```python
from build123d import *

# Parameters (mm, degrees)
SKETCH1_W           = 15
SKETCH1_H           = 4
BOSS_EXTRUDE1_DEPTH = 4.5
SKETCH2_W           = 6
SKETCH2_H           = 3
CUT_EXTRUDE1_DEPTH  = 4.5
SKETCH3_W           = 0.5
SKETCH3_H           = 4.5
CUT_EXTRUDE2_DEPTH  = 9.5
SKETCH4_W           = 0.5
SKETCH4_H           = 4.5
CUT_EXTRUDE3_DEPTH  = 9.5
SKETCH6_W           = 14
SKETCH6_H           = 0.5
CUT_EXTRUDE5_DEPTH  = 9.5


with BuildPart() as part:
    # Sketch1 → Boss-Extrude1 (new body)
    with BuildSketch(Plane(origin=(0, 0, 0), x_dir=(1, 0, 0), z_dir=(0, 1, 0))):
        with Locations((7.5, 2)):
            Rectangle(SKETCH1_W, SKETCH1_H)
    extrude(amount=BOSS_EXTRUDE1_DEPTH)

    # Sketch2 → Cut-Extrude1 (cut)
    with BuildSketch(Plane(origin=(0, 4.5, 0), x_dir=(1, 0, 0), z_dir=(0, 1, 0))):
        with Locations((7.5, 2.5)):
            Rectangle(SKETCH2_W, SKETCH2_H)
    extrude(amount=-CUT_EXTRUDE1_DEPTH, mode=Mode.SUBTRACT)

    # Sketch3 → Cut-Extrude2 (cut)
    with BuildSketch(Plane(origin=(0, 0, -4), x_dir=(-1, 0, 0), z_dir=(0, 0, -1))):
        with Locations((-0.25, 2.25)):
            Rectangle(SKETCH3_W, SKETCH3_H)
    extrude(amount=-CUT_EXTRUDE2_DEPTH, mode=Mode.SUBTRACT)

    # Sketch4 → Cut-Extrude3 (cut)
    with BuildSketch(Plane(origin=(0, 0, -4), x_dir=(-1, 0, 0), z_dir=(0, 0, -1))):
        with Locations((-14.75, 2.25)):
            Rectangle(SKETCH4_W, SKETCH4_H)
    extrude(amount=-CUT_EXTRUDE3_DEPTH, mode=Mode.SUBTRACT)

    # Sketch6 → Cut-Extrude5 (cut)
    with BuildSketch(Plane.XY):
        with Locations((7.5, 4.25)):
            Rectangle(SKETCH6_W, SKETCH6_H)
    extrude(amount=-CUT_EXTRUDE5_DEPTH, mode=Mode.SUBTRACT)


solid = part.part
```
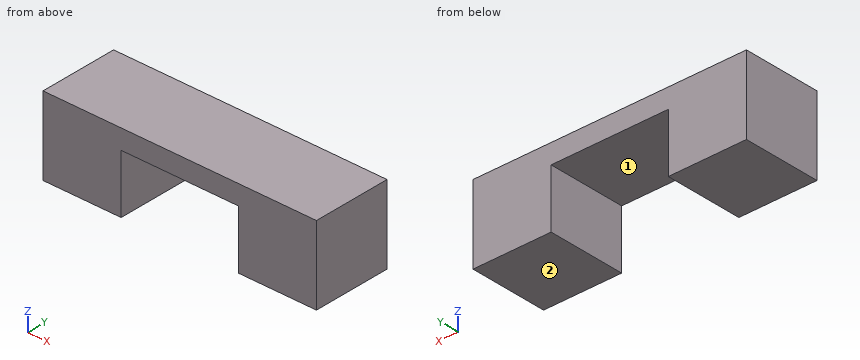
Input: part model. Units: mm. Frame: model coordinates. Face numbers are marked on the shaded views. A direction names the side the tool comes from. Give positions to 0.01 mm unless a question says otherwise; leave off trailing zeros. Order: outer loops, then holes, each group sorted by start corner. A loop starts at its lowest first (then second) coordinate and runs counter-clockwise, first axis right, second up.
1. Pin query (flat end, axial travel): pin 1 Ø1.5 at (x, y) = (9, 3) entering from +Z; pin 2 Ø2 at (x, y) = (8.5, 3) entering from -Z. Return the tip coordinate at first contact, or that it passes through.
Computed:
pin 1: stops at z = 0
pin 2: stops at z = -1
2. Cut plane A-A (z = -2.2). Return loops of the section in (x, y), and give its area (3 significant figures).
Computed:
outline: (0.5, 0) - (4.5, 0) - (4.5, 4) - (0.5, 4) - close; (10.5, 0) - (14.5, 0) - (14.5, 4) - (10.5, 4) - close
area: 32.0 mm2
3. Cut plane C-C (x = 5). Return loops of the section in (y, z).
Computed:
outline: (0, -1) - (4, -1) - (4, 0) - (0, 0) - close
4. Set-up query: the marked faces 1 and 2. Return all of +Z, -Z, +X, -X, +Y, -Y with unobstructed straight access to the full face (end or side cutting, diameter ignored); none if empty.
Computed:
face 1: -Z, +Y, -Y
face 2: -Z, +X, -X, +Y, -Y
5. Cut plane B-B (y = 1.9). Return loops of the section in (x, z), and give its area (3 significant figures).
Computed:
outline: (0.5, -4) - (4.5, -4) - (4.5, -1) - (10.5, -1) - (10.5, -4) - (14.5, -4) - (14.5, 0) - (0.5, 0) - close
area: 38.0 mm2
6. Line query: probe 1 along X at (y, z) = (2.4, -1.2); probe 2 along Z at (x, y) = (8, 3.7). Output: solid intervals per line, ascending.
Computed:
probe 1: x = 0.5 to 4.5, 10.5 to 14.5
probe 2: z = -1 to 0
